```python
from build123d import *

# Parameters (mm, degrees)
CROQUIS1_W              = 30
CROQUIS1_H              = 30
CROQUIS1_R              = 1
SALIENTE_EXTRUIR2_DEPTH = 1
CROQUIS2_W              = 30
CROQUIS2_H              = 30
CROQUIS2_W_2            = 24
CROQUIS2_H_2            = 24
SALIENTE_EXTRUIR3_DEPTH = 10


with BuildPart() as part:
    # Croquis1 → Saliente-Extruir2 (new body)
    with BuildSketch(Plane.XY.offset(0.6)):
        Rectangle(CROQUIS1_W, CROQUIS1_H)
        with Locations((-8, 0)):
            Circle(CROQUIS1_R, mode=Mode.SUBTRACT)
        with Locations((8, 0)):
            Circle(CROQUIS1_R, mode=Mode.SUBTRACT)
        with BuildLine():
            Line((-1.75, 4.25), (1.75, 4.25))
            ThreePointArc((1.75, 4.25), (6, 0), (1.75, -4.25))
            Line((1.75, -4.25), (-1.75, -4.25))
            ThreePointArc((-1.75, -4.25), (-6, 0), (-1.75, 4.25))
        make_face(mode=Mode.SUBTRACT)
    extrude(amount=-SALIENTE_EXTRUIR2_DEPTH)

    # Croquis2 → Saliente-Extruir3 (add)
    with BuildSketch(Plane.XY.offset(0.6)):
        Rectangle(CROQUIS2_W, CROQUIS2_H)
        Rectangle(CROQUIS2_W_2, CROQUIS2_H_2, mode=Mode.SUBTRACT)
    extrude(amount=SALIENTE_EXTRUIR3_DEPTH)


solid = part.part
```
CAD build for the part. Positions are in the model's coordinates, mm. A direction names the side the tool comes from. Coordinates: 2 decimals unless noted, no trailing zeros. Order: outer loops, then holes, each group sorted by start corner. A loop starts at its lowest first (then second) coordinate and runs counter-clockwise, first axis right, second up. Notation, with made-up numbers: (3, 88) - (35, 88) arc R32 cw to (35, 116) - close; hole circle Ø6 at (-18.5, 48.25). An arc over 180 degrees is marked (long way). Use a Markdown table: item, result. Add a question column.
(1) Drill centre lines: line 1 along X through (y, z) = (-9.5, 6.25); line 2 along Y through (x, z) = (8, 0.05). Where is each one in solid material? Low to high. Write a range as [from, to].
(2) Which spindle directions (+Z, -Z, +X, -X, +Y, -Y) get a long thin tool onto all of the face, cutting with end or side? Do faces 4 (the face through (0, 4.25, 0)), 5 (the face through (0, 12, 6)), 6 (the face through (0, 7, -0.4)). Say none if no direction does.
(3) Saw through at C-C (y = 0). Give the cut face in (x, z), then the cut area to 3 significant figures.
(4) Saw through at B-B (z = 2). Give the cut face in (x, y).
(5) Saw through at A-A (x = 8). Give the cut face in (y, z), then the cut area to 3 significant figures.
(6) Pull direction Y, two halves, no side cores. Call faces 1 (the face through (0, 6, 0.6)), 2 (the face through (0, 15, 5)), 3 (the face through (-15, 0, 5)): +Y half, -Y half, draft (parallel to the pull), parting line (faces both ways), or undercut.
(7) Saw through at D-D (y = -8.5). Give the cut face in (x, z), then the cut area to 3 significant figures.
(8) Flat gauge pin, fed straight in: pin 1 (3 mm diameter, centred on x = -3.5, y = -9.5, fed in from +Z). Where does the tip first touch, or does it go through?
Solved:
| question | item | result |
|---|---|---|
| 1 | line 1 | x = [-15, -12], [12, 15] |
| 1 | line 2 | y = [-15, -1], [1, 15] |
| 2 | face 4 | +Z, -Z |
| 2 | face 5 | +Z |
| 2 | face 6 | -Z, +X, -X, +Y, -Y |
| 3 | outline | (-15, -0.4) - (-9, -0.4) - (-9, 0.6) - (-12, 0.6) - (-12, 10.6) - (-15, 10.6) - close; (-7, -0.4) - (-6, -0.4) - (-6, 0.6) - (-7, 0.6) - close; (6, -0.4) - (7, -0.4) - (7, 0.6) - (6, 0.6) - close; (9, -0.4) - (15, -0.4) - (15, 10.6) - (12, 10.6) - (12, 0.6) - (9, 0.6) - close |
| 3 | area | 74.0 mm² |
| 4 | outline | (-15, -15) - (15, -15) - (15, 15) - (-15, 15) - close; hole (-12, -12) - (12, -12) - (12, 12) - (-12, 12) - close |
| 5 | outline | (-15, -0.4) - (-1, -0.4) - (-1, 0.6) - (-12, 0.6) - (-12, 10.6) - (-15, 10.6) - close; (1, -0.4) - (15, -0.4) - (15, 10.6) - (12, 10.6) - (12, 0.6) - (1, 0.6) - close |
| 5 | area | 88.0 mm² |
| 6 | face 1 | undercut |
| 6 | face 2 | +Y half |
| 6 | face 3 | draft |
| 7 | outline | (-15, -0.4) - (15, -0.4) - (15, 10.6) - (12, 10.6) - (12, 0.6) - (-12, 0.6) - (-12, 10.6) - (-15, 10.6) - close |
| 7 | area | 90.0 mm² |
| 8 | pin 1 | stops at z = 0.6 |
